from build123d import *

# Parameters (mm, degrees)
F1_DEPTH = 15
F2_R     = 1.25
F3_DEPTH = 25
F4_R     = 1
F5_DEPTH = 35.201
F6_R     = 3
F7_R     = 11


with BuildPart() as f1:
    # F0 (on Top) → F1 (new body)
    with BuildSketch(Plane.XY):
        with BuildLine():
            Line((1.6, 0), (0, 0))
            Line((0, 0), (0, -21.6))
            Line((0, -21.6), (35.2, -21.6))
            Line((35.2, -21.6), (35.2, 0))
            Line((35.2, 0), (33.6, 0))
            Line((33.6, 0), (33.6, -17))
            ThreePointArc((33.6, -17), (32.72132, -19.12132), (30.6, -20))
            Line((30.6, -20), (4.6, -20))
            ThreePointArc((4.6, -20), (2.47868, -19.12132), (1.6, -17))
            Line((1.6, -17), (1.6, 0))
        make_face()
    extrude(amount=F1_DEPTH)

    # F2 (on face) → F3 (cut)
    with BuildSketch(Plane.XZ.offset(21.6)):
        with Locations((2.85, 3)):
            Circle(F2_R)
        with Locations((32.35, 3)):
            Circle(F2_R)
    extrude(amount=-F3_DEPTH, mode=Mode.SUBTRACT)

    # F4 (on face) → F5 (cut, through all)
    with BuildSketch(Plane.YZ.offset(35.2)):
        with Locations((-3.6, 12)):
            Circle(F4_R)
    extrude(amount=-F5_DEPTH, mode=Mode.SUBTRACT)

    # F6
    f6_edges = [f1.edges().sort_by_distance(p)[0] for p in [
        (0.8, 0, 15),
        (34.4, 0, 15),
    ]]
    fillet(f6_edges, radius=F6_R)

    # F7
    f7_edges = [f1.edges().sort_by_distance(p)[0] for p in [
        (34.4, 0, 0),
        (0.8, 0, 0),
    ]]
    fillet(f7_edges, radius=F7_R)


solid = f1.part
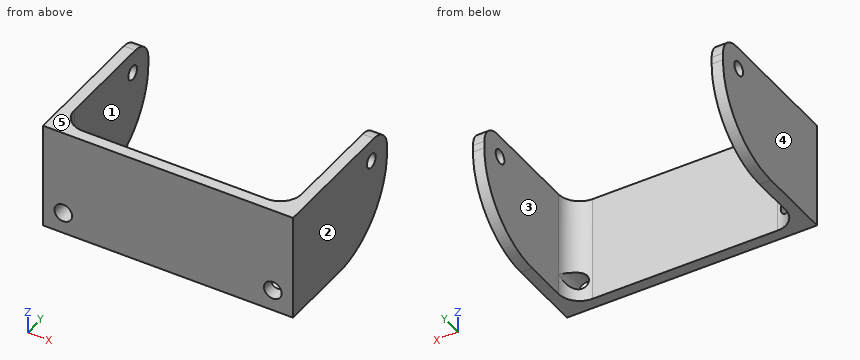
Model file for the job. Use its own axes, mm. Face numbers are marked on the shaded views. A direction names the side the tool comes from. Give positions to 0.01 mm unless a question says otherwise; leave off trailing zeros. Order: outer loops, then holes, each group sorted by start corner. A loop starts at its lowest first (then second) coordinate and runs counter-clockwise, first axis right, second up. Notation, with made-up numbers: (70.5, 85) - (115.5, 85) arc R25 cw to (115.5, 105) - close; hole circle Ø5 at (-24, 53). An arc over 180 degrees is marked (long way). One line per item, written item: value.
Item 1: Slice it at B-B (x = 2.85). List the corners of the cut face in (y, z), then the cut area to 3 significant figures.
Response values:
outline: (-21.6, 0) - (-19.44, 0) - (-19.44, 1.75) - (-21.6, 1.75) - close; (-21.6, 4.25) - (-19.44, 4.25) - (-19.44, 15) - (-21.6, 15) - close
area: 27.0 mm2
Item 2: Pin check, flat tips, straight feed: pin 1 Ø3 at (x, z) = (32.35, 3) entering from +Y; pin 2 Ø4.5 at (x, z) = (15, 10) entering from +Y. Stop position of each tip, or through.
Response values:
pin 1: y = -2.66
pin 2: y = -20
Item 3: Slice it at D-D (z = 14). List the corners of the cut face in (x, y), then the cut area to 3 significant figures.
Response values:
outline: (0, -21.6) - (35.2, -21.6) - (35.2, -0.76) - (33.6, -0.76) - (33.6, -17) arc R3 cw to (30.6, -20) - (4.6, -20) arc R3 cw to (1.6, -17) - (1.6, -0.76) - (0, -0.76) - close
area: 122 mm2
Item 4: Tool access for the marked faces 1 and 2: list every direction of +Z, -Z, +X, -X, +Y, -Y with a clear straight run to the whole face (end or side of a thin tool).
Response values:
face 1: +Z, -Z, +Y
face 2: +Z, -Z, +X, +Y, -Y
Item 5: Wall check: line 1 (X direction, y = -5, z = 9); line 2 (Z direction, x = 32.35, y = -19.55); line 3 (Y direction, x = 28, z = 8.25). Give the ranges that are in metal, low to high.
Response values:
line 1: 0 to 1.6, 33.6 to 35.2
line 2: 0 to 1.75, 4.25 to 15
line 3: -21.6 to -20
Item 6: Slice it at A-A (y = -16.25). List the corners of the cut face in (x, z), then the cut area to 3 significant figures.
Response values:
outline: (0, 0) - (1.6, 0) - (1.6, 15) - (0, 15) - close; (33.6, 0) - (35.2, 0) - (35.2, 15) - (33.6, 15) - close
area: 48.0 mm2
Item 7: Slice it at C-C (y = -3.6). List the corners of the cut face in (x, z), then the cut area to 3 significant figures.
Response values:
outline: (0, 2.86) - (1.6, 2.86) - (1.6, 11) - (0, 11) - close; (0, 13) - (1.6, 13) - (1.6, 15) - (0, 15) - close; (33.6, 2.86) - (35.2, 2.86) - (35.2, 11) - (33.6, 11) - close; (33.6, 13) - (35.2, 13) - (35.2, 15) - (33.6, 15) - close
area: 32.4 mm2
Item 8: Two-plate mould, pull along X, no slides. Class the marked faces 3, 4 and 5: released by +X, released by -X, zero draft, split by the parting line, or undercut.
Response values:
face 3: undercut
face 4: released by -X
face 5: zero draft
